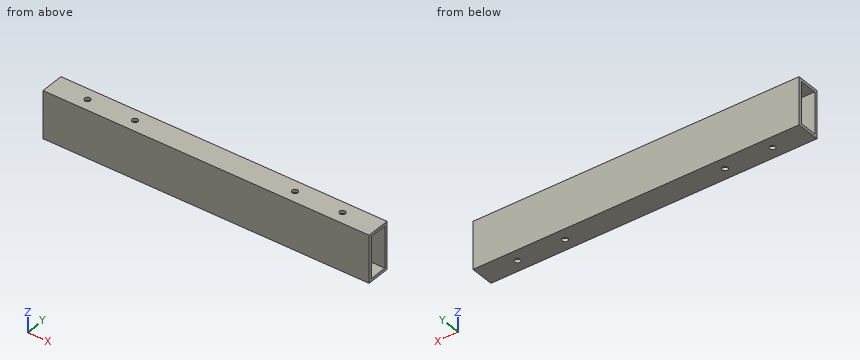
Autodesk Inventor part; units mm, degrees
ref_plane "YZ Plane" through (0, 0, 0) normal (1, 0, 0) x (0, 1, 0)
ref_plane "XZ Plane" through (0, 0, 0) normal (0, 1, 0) x (-1, 0, 0)
ref_plane "XY Plane" through (0, 0, 0) normal (0, 0, 1) x (1, 0, 0)
sketch "Sketch1" plane through (0, 0, 0) normal (0, 1, 0) x (-1, 0, 0)
  line L0 (0, 0) -> (349.25, 0)
  line L1 (349.25, 0) -> (349.25, 50.8)
  line L2 (349.25, 50.8) -> (0, 50.8)
  line L3 (0, 50.8) -> (0, 0)
  dimension "d0" = 349.25
  dimension "d1" = 50.8
extrude "Extrusion1" add sketch "Sketch1" along normal blind 25.4
sketch "Sketch2" plane through (0, 0, 50.8) normal (1, 0, 0) x (0, 0, -1)
  line L0 (0, 25.4) -> (3.175, 25.4)
  line L1 (3.175, 25.4) -> (3.175, 22.225)
  line L2 (3.175, 22.225) -> (0, 22.225)
  line L3 (0, 22.225) -> (0, 25.4)
  line L4 (3.175, 22.225) -> (47.625, 22.225)
  line L5 (47.625, 22.225) -> (47.625, 3.175)
  line L6 (47.625, 3.175) -> (3.175, 3.175)
  line L7 (3.175, 3.175) -> (3.175, 22.225)
  dimension "d4" = 3.175
  dimension "d5" = 3.175
  dimension "d6" = 44.45
  dimension "d7" = 19.05
extrude "Extrusion2" cut sketch "Sketch2" against normal blind 508 contours L4 L5 L6 L7
sketch "Sketch3" plane through (-349.25, 0, 50.8) normal (0, 0, 1) x (1, 0, 0)
  line L0 (349.25, 0) -> (349.25, 25.4)
  line L1 (0, 0) -> (0, 25.4)
  line L2 (0, 12.7) -> (38.1, 12.7)
  line L3 (0, 12.7) -> (38.1, 12.7) construction
  line L4 (38.1, 12.7) -> (88.9, 12.7)
  circle A0 centre (88.9, 12.7) radius 3.175
  circle A1 centre (38.1, 12.7) radius 3.175
  line L5 (349.25, 12.7) -> (311.15, 12.7)
  line L6 (349.25, 12.7) -> (387.35, 12.7) construction
  line L7 (311.15, 12.7) -> (260.35, 12.7)
  line L8 (311.15, 12.7) -> (361.95, 12.7) construction
  circle A2 centre (260.35, 12.7) radius 3.175
  circle A3 centre (311.15, 12.7) radius 3.175
  dimension "d10" = 38.1
  dimension "d11" = 0
  dimension "d12" = 50.8
  dimension "d13" = 180
  dimension "d14" = 6.35
  dimension "d15" = 6.35
  dimension "d16" = 38.1
  dimension "d17" = 180
  dimension "d18" = 50.8
  dimension "d19" = 180
  dimension "d20" = 6.35
  dimension "d21" = 6.35
extrude "Extrusion3" cut sketch "Sketch3" against normal blind 50.8
properties part number "CatapultMotorSupport"
Here's how the part is built. I have some questions about the finished solid (model axes, mm). Give positions to 0.01 mm unless a question says otherwise; leave off trailing zeros. Write each loop counter-clockwise with the first axis right and the second up, starting at its lowest first coordinate (ties: lowest second). Pieces come first, ordered by that corner, then holes.
(1) Imagine slicing it at B-B, the plane z = 18. Write out the boundary of the cut face in (x, y) (3 decimals).
Output values:
outline: (-349.25, 0) - (0, 0) - (0, 3.175) - (-349.25, 3.175) - close; (-349.25, 22.225) - (0, 22.225) - (0, 25.4) - (-349.25, 25.4) - close
(2) Imagine slicing it at A-A, the plane x = -21.5. Write out the boundary of the cut face in (y, z) (3 decimals).
Output values:
outline: (0, 0) - (25.4, 0) - (25.4, 50.8) - (0, 50.8) - close; hole (3.175, 3.175) - (22.225, 3.175) - (22.225, 47.625) - (3.175, 47.625) - close
(3) Imagine slicing it at C-C, the plane y = 12.7. Count the separate pieces of the cut face and the enclosed holes in it, and give its area (3 significant figures).
Output values:
separate pieces: 10
enclosed holes: 0
area: 2,060 mm2
(4) If I drill on L1, parallel to Z at x = -25, y = 8.5 (3 decimals); L2, parallel to Y at x = -184, z = 32.5 (3 decimals); L3, parallel to Y at x = -311.15, z = 48.45 (3 decimals), over which ranges is the centre line in solid material (lowest first)?
Output values:
L1: z = 0 to 3.175, 47.625 to 50.8
L2: y = 0 to 3.175, 22.225 to 25.4
L3: y = 0 to 9.525, 15.875 to 25.4
